Source: CAD feature listing. Evaluate the final solid. Frame: model axes, mm. Face numbers are marked on the shaded views. A direction names the side the tool comes from. Round coordinates to 2 decimals unless told otherwise and drop trailing zeros. Order: outer loops, then holes, each group sorted by start corner. A loop starts at its lowest first (then second) coordinate and runs counter-clockwise, first axis right, second up. Notation, with made-up numbers: (-32, 87.5) - (-27, 87.5) arc R17 cw to (-27, 109.5) - close; hole circle Ø7 at (-24, -5). An arc over 180 degrees is marked (long way). Put each result on its own line as item: value. Start each with the question number.
1) Section C-C on x = 30.5. Output: boundary loops of the cut face in (y, z).
2) Mould query, pull axis X, two halves, no side actions, for the marked faces 1, 2 and 3. Classes: +X half, -X half, draft (parallel to the pull), parting line (faces both ways), or undercut.
3) Line query: probe 1 along Y at (x, z) = (-18, -40.5); probe 2 along Z at (x, y) = (19.5, 7.5); probe 3 along X at (y, z) = (-12.5, -60). Output: solid intervals per line, ascending. Write a range as [from, to].
4) Contact query for flat-ended pins moving along their axis: P1, Ø4, axis at x = -14.5, z = -44.5, coming from the +Y side; P2, Ø11, axis at x = -38.33, y = -22.5, coming from the +Z side; P3, Ø12, axis at y = 27.5, z = -54, coming from the +X side; P4, Ø5, axis at y = -17, z = -10.5, coming from the +X side. Output: stop coordinate, or through.
5) Section B-B on z = -55. Output: boundary loops of the cut face in (x, y), then the cut area to 3 significant figures.
6) Section D-D on y = 0. Output: boundary loops of the cut face in (x, z), then the cut area to 3 significant figures.
7) Section A-A on y = -22.5. Output: boundary loops of the cut face in (x, z), then the cut area to 3 significant figures.
8) Access query for the marked faces 4, 5 and 6. Directions: +Z, -Z, +X, -X, +Y, -Y. A direction counts if a zero-diameter tool reaches every point of the face in a straight line with its end or side. Return the directions, or none.
```python
from build123d import *

# Parameters (mm, degrees)
F2_DEPTH = 37.5
F3_DEPTH = 6
F0_R     = 18
F0_R_2   = 11
F4_DEPTH = 25
F0_R_3   = 6
F5_DEPTH = 63.001


with BuildPart() as f2:
    # F1 (on Front) → F2 (new body, symmetric)
    with BuildSketch(Plane.XZ):
        Polygon((-66.326725, -48), (-66.326725, -63), (-54.326725, -63), (-54.326725, -58), (-22.326725, -58), (-22.326725, -63), (-10.326725, -63), (-10.326725, -48), align=None)
    extrude(amount=F2_DEPTH, both=True)

    # F1 (on Front) → F3 (join, symmetric)
    with BuildSketch(Plane.XZ):
        Polygon((-2.326725, 0), (-66.326725, -48), (-10.326725, -48), (-10.326725, -63), (16.690247, -25), (16.690247, 0), align=None)
    extrude(amount=F3_DEPTH, both=True)

    # F0 (on Top) → F4 (join)
    with BuildSketch(Plane.XY):
        with Locations((33.673275, 0)):
            Circle(F0_R)
        with Locations((33.673275, 0)):
            Circle(F0_R_2, mode=Mode.SUBTRACT)
    extrude(amount=-F4_DEPTH)

    # F0 (on Top) → F5 (cut, through all)
    with BuildSketch(Plane.XY):
        with Locations((-38.326725, 22.5)):
            Circle(F0_R_3)
        with Locations((-38.326725, -22.5)):
            Circle(F0_R_3)
    extrude(amount=-F5_DEPTH, mode=Mode.SUBTRACT)


solid = f2.part
```
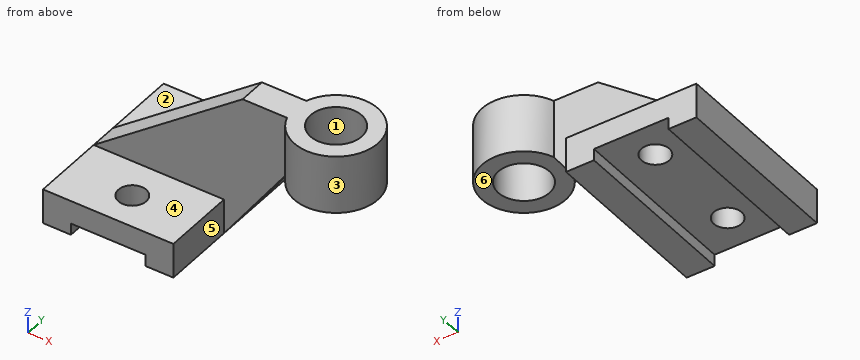
Answer sheet:
1. outline: (-17.72, -25) - (-10.53, -25) - (-10.53, 0) - (-17.72, 0) - close; (10.53, -25) - (17.72, -25) - (17.72, 0) - (10.53, 0) - close
2. face 1: undercut
2. face 2: draft
2. face 3: parting line
3. probe 1: [-6, 6]
3. probe 2: [-25, 0]
3. probe 3: [-66.33, -54.33], [-22.33, -10.33]
4. P1: y = 6
4. P2: through
4. P3: x = -10.33
4. P4: x = 44.34
5. outline: (-66.33, -37.5) - (-10.33, -37.5) - (-10.33, -6) - (-4.64, -6) - (-4.64, 6) - (-10.33, 6) - (-10.33, 37.5) - (-66.33, 37.5) - close; hole circle Ø12 at (-38.33, -22.5); hole circle Ø12 at (-38.33, 22.5)
5. area: 4,040 mm^2
6. outline: (-66.33, -63) - (-54.33, -63) - (-54.33, -58) - (-22.33, -58) - (-22.33, -63) - (-10.33, -63) - (16.69, -25) - (22.67, -25) - (22.67, 0) - (-2.33, 0) - (-66.33, -48) - close; (44.67, -25) - (51.67, -25) - (51.67, 0) - (44.67, 0) - close
6. area: 3,350 mm^2
7. outline: (-66.33, -63) - (-54.33, -63) - (-54.33, -58) - (-44.33, -58) - (-44.33, -48) - (-66.33, -48) - close; (-32.33, -58) - (-22.33, -58) - (-22.33, -63) - (-10.33, -63) - (-10.33, -48) - (-32.33, -48) - close
7. area: 560 mm^2
8. face 4: +Z, +X, -X, -Y
8. face 5: +Z, -Z, +X, -Y
8. face 6: -Z, +X, +Y, -Y
